Drawing for the job (mm, zero at the part's lowest x, y, z). Round coordinates to 2 decimals unless told otherwise and drop trailing zeros. Order: outer loops, then holes, each group sorted by start corner. A loop starts at its lowest first (then second) coordinate and runs counter-clockwise, first axis right, second up. Notation, with made-up numbers: (5, -1) - (16, -1) arc R19 ccw to (16, 14) - close; hole circle Ø11 at (11.5, 37). An arc over 180 degrees is marked (long way). Answer as a JSON object with one key per item and string values.
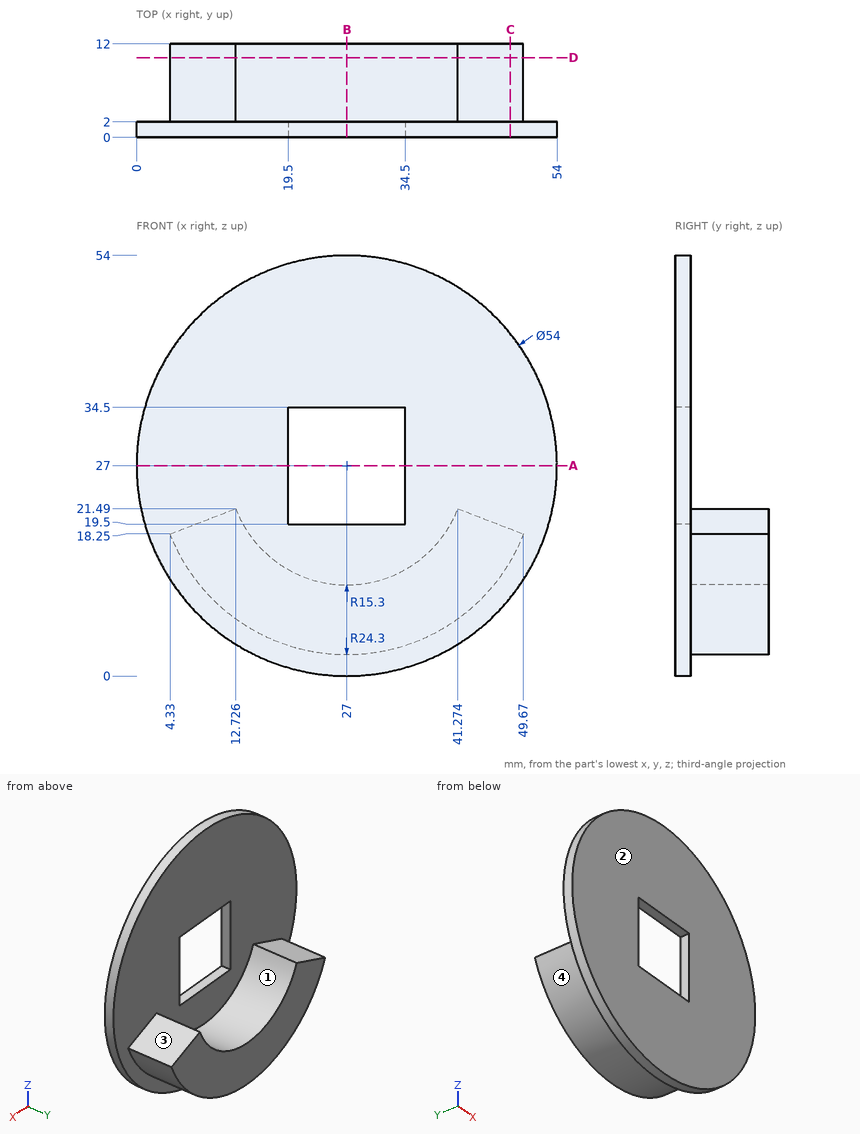
Item 1: Drop flat-ended pins along their axis: P1, Ø4, axis at x = 37, y = 9, coming from the +Z side; P2, Ø2, axis at x = 28, y = 1, coming from the -Z side; P3, Ø0.6, axis at y = 1.5, z = 29.5, coming from the -X side; P4, Ø0.6, axis at y = 1, z = 24.5, coming from the +X side. Give the stop position or say it passes through.
Taken from the geometry:
{"P1": "z = 17.51", "P2": "z = 0", "P3": "x = 0.09", "P4": "x = 53.91"}
Item 2: Probe L1, parallel to Y at x = 49.5, z = 15.5; L2, parallel to Z at x = 26.5, y = 4.75 (1 decimal); L3, parallel to X at y = 6.5, z = 14 (1 decimal). List the from-to ranges inside material, lowest first. Write a range as from..to.
Taken from the geometry:
{"L1": "0..2", "L2": "2.7..11.7", "L3": "6.5..18.9, 35.1..47.5"}
Item 3: Cut at C-C (x = 48). Write the cut outline in (y, z), plus the area to 3 significant figures.
Taken from the geometry:
{"outline": "(0, 10.03) - (2, 10.03) - (2, 14.77) - (12, 14.77) - (12, 18.89) - (2, 18.89) - (2, 43.97) - (0, 43.97) - close", "area": "109 mm2"}
Item 4: Cut at A-A (z = 27). Write the cut outline in (x, y).
Taken from the geometry:
{"outline": "(0, 0) - (19.5, 0) - (19.5, 2) - (0, 2) - close; (34.5, 0) - (54, 0) - (54, 2) - (34.5, 2) - close"}
Item 5: Two-plate mould, pull along X, no slides. Class the marked faces 1, 2, 3 and 4: pulls with the +X half, pulls with the -X half, needs draft (parallel to the pull), parting line crosses it, or undercut.
Taken from the geometry:
{"face 1": "undercut", "face 2": "needs draft", "face 3": "pulls with the +X half", "face 4": "parting line crosses it"}
Item 6: Cut at D-D (y = 10.25). Write the cut outline in (x, z).
Taken from the geometry:
{"outline": "(4.33, 18.25) arc R24.3 ccw to (49.67, 18.25) - (41.27, 21.49) arc R15.3 cw to (12.73, 21.49) - close"}
Item 7: Cut at B-B (x = 27). Write the cut outline in (y, z).
Taken from the geometry:
{"outline": "(0, 0) - (2, 0) - (2, 2.7) - (12, 2.7) - (12, 11.7) - (2, 11.7) - (2, 19.5) - (0, 19.5) - close; (0, 34.5) - (2, 34.5) - (2, 54) - (0, 54) - close"}
